CAD build for the part. Positions are in the model's coordinates, mm. A direction names the side the tool comes from. Give positions to 0.01 mm unless a question says otherwise; leave off trailing zeros. Loops run counter-clockwise (first coordinate to the right, second up) from the corner with the lowest first, then second, coordinate; pieces in that order, holes last.
Item 1: Which spindle directions (+Z, -Z, +X, -X, +Y, -Y) get a long thin tool onto all of the face, cutting with end or side? Do faces 1 (the flat face through (13, 0, 13)), 2 (the flat face through (0, 25.8, 7)), 3 (the cylindrical face through (14, 12.3, 2.6)). Say none if no direction does.
Item 2: Mould opens along Z. For faces 4 (the cylindrical face through (14.01, -15.39, 22.49)), 5 (the flat face through (-13.4, 2.1, 0)), 6 (the flat face through (15, 0, 13)) say: released by +Z, released by -Z, zero draft, split by the parting line, or undercut.
Item 3: Saw through at C-C on z = 13.5. Give the cut face in (x, y).
Item 4: Probe probe 1 along Y at (x, z) = (14.5, 23.5); probe 2 along Z at (x, y) = (14.25, -16.5); probe 3 along X at (y, z) = (18.5, 20). List the from-to ranges inside material, lowest first.
Item 5: Saw through at A-A on x = 9.5. Give the cut face in (y, z).
Item 6: Saw through at B-B on y = -2.5. Give the cut face in (x, z), plus the area to 3 significant figures.
Item 7: Drop flat-ended pins along their axis: P1, Ø14, axis at x = 0, z = 13.5, coming from the -Y side; P2, Ø3, axis at x = -6, z = 20, coming from the +Y side. Give the stop position or say it passes through.
Item 8: Saw through at D-D on y = -16.5. Give the cut face in (x, z), plus the area to 3 significant figures.
from build123d import *

# Parameters (mm, degrees)
SKETCH_2_W          = 30
SKETCH_2_H          = 53
SKETCH_2_W_2        = 26
SKETCH_2_H_2        = 49
EXTRUDE_1_DEPTH     = 27
SKETCH_3_W          = 26
SKETCH_3_H          = 27
CUT_EXTRUDE_1_DEPTH = 0.7
SKETCH_4_R          = 3.5
CUT_EXTRUDE_2_DEPTH = 38
SKETCH_5_R          = 1.5
CUT_EXTRUDE_3_DEPTH = 3
SKETCH_6_R          = 6
CUT_EXTRUDE_4_DEPTH = 3


with BuildPart() as part:
    # 草图2 → 拉伸-薄壁1 (new body)
    with BuildSketch(Plane.XY):
        Rectangle(SKETCH_2_W, SKETCH_2_H)
        Rectangle(SKETCH_2_W_2, SKETCH_2_H_2, mode=Mode.SUBTRACT)
    extrude(amount=EXTRUDE_1_DEPTH)

    # 草图3 → 切除-拉伸1 (cut)
    with BuildSketch(Plane(origin=(0, 26.5, 0), x_dir=(1, 0, 0), z_dir=(0, 1, 0))):
        with Locations((0, -13.5)):
            Rectangle(SKETCH_3_W, SKETCH_3_H)
    extrude(amount=-CUT_EXTRUDE_1_DEPTH, mode=Mode.SUBTRACT)

    # 草图4 → 切除-拉伸2 (cut)
    with BuildSketch(Plane.XZ.offset(26.5)):
        with Locations(Location((0, 13.5, 0), (0, 0, 270))):
            Circle(SKETCH_4_R)
    extrude(amount=-CUT_EXTRUDE_2_DEPTH, mode=Mode.SUBTRACT)

    # 草图5 → 切除-拉伸3 (cut)
    with BuildSketch(Plane(origin=(15, 0, 0), x_dir=(0, 0, -1), z_dir=(1, 0, 0))):
        with Locations(Location((-3.5, -16.5, 0), (0, 0, 90))):
            Circle(SKETCH_5_R)
        with Locations(Location((-3.5, 13.5, 0), (0, 0, 90))):
            Circle(SKETCH_5_R)
        with Locations(Location((-23.5, -16.5, 0), (0, 0, 270))):
            Circle(SKETCH_5_R)
        with Locations(Location((-23.5, 13.5, 0), (0, 0, 270))):
            Circle(SKETCH_5_R)
    extrude(amount=-CUT_EXTRUDE_3_DEPTH, mode=Mode.SUBTRACT)

    # 草图6 → 切除-拉伸4 (cut)
    with BuildSketch(Plane(origin=(0, 25.8, 0), x_dir=(1, 0, 0), z_dir=(0, 1, 0))):
        with Locations(Location((0, -13.5, 0), (0, 0, 270))):
            Circle(SKETCH_6_R)
    extrude(amount=-CUT_EXTRUDE_4_DEPTH, mode=Mode.SUBTRACT)


solid = part.part
Results below:
1. face 1: +Z, -Z
1. face 2: +Z, -Z, +Y
1. face 3: +X
2. face 4: undercut
2. face 5: released by -Z
2. face 6: zero draft
3. outline: (-15, -26.5) - (-3.5, -26.5) - (-3.5, -24.5) - (-13, -24.5) - (-13, 24.5) - (-6, 24.5) - (-6, 25.8) - (-13, 25.8) - (-13, 26.5) - (-15, 26.5) - close; (3.5, -26.5) - (15, -26.5) - (15, 26.5) - (13, 26.5) - (13, 25.8) - (6, 25.8) - (6, 24.5) - (13, 24.5) - (13, -24.5) - (3.5, -24.5) - close
4. probe 1: y = -26.5 to -18, -15 to 12, 15 to 26.5
4. probe 2: z = 0 to 2, 5 to 22, 25 to 27
4. probe 3: x = -15 to -13, 13 to 15
5. outline: (-26.5, 0) - (-24.5, 0) - (-24.5, 27) - (-26.5, 27) - close; (24.5, 0) - (25.8, 0) - (25.8, 27) - (24.5, 27) - close
6. outline: (-15, 0) - (-13, 0) - (-13, 27) - (-15, 27) - close; (13, 0) - (15, 0) - (15, 27) - (13, 27) - close
6. area: 108 mm2
7. P1: stops at y = -26.5
7. P2: stops at y = 25.8
8. outline: (-15, 0) - (-13, 0) - (-13, 27) - (-15, 27) - close; (13, 0) - (15, 0) - (15, 2) - (13, 2) - close; (13, 5) - (15, 5) - (15, 22) - (13, 22) - close; (13, 25) - (15, 25) - (15, 27) - (13, 27) - close
8. area: 96.0 mm2
